Part model, mm, in its own coordinate system. A direction names the side the tool comes from. Give positions to 0.01 mm unless a question says otherwise; leave off trailing zeros. Write each loop counter-clockwise with the first axis right and the second up, starting at its lowest first coordinate (ties: lowest second). Pieces come first, ordered by that corner, then holes. Notation, with made-up numbers: M -7.75,-3.5 L 28.25,-3.5 A25 cw 28.25,13.5 Z; hole C 51.25,-32 d2. An arc over 180 degrees is marked long. Answer as CSV lines item,"result". Start each with the question number.
1) Mould opens along X. For faces 4 (the flat face through (0, 24.3, 2)), 5 (the flat face through (-31, 8, 2)), 6 (the flat face through (-8, -21, 2)) say: pulls with the +X half, pulls with the -X half, needs draft (parallel to the pull), parting line crosses it, or undercut.
2) Pin check, flat tips, straight feed: pin 1 Ø1.6 at (y, z) = (-22.5, 2) entering from -X; pin 2 Ø1 at (y, z) = (8.5, 2.5) entering from +X; pin 3 Ø1.6 at (x, z) = (-9, 1.5) entering from -Y. Stop position of each tip, or through.
3) Wall check: line 1 along X through (y, z) = (-22, 2.9); line 2 along Y through (x, z) = (11, 0.25); line 3 along X through (y, z) = (-5, 1.25). Give the ranges that are in metal, low to high. Write a range as from..to.
4) Slice it at B-B, the plane x = -26. Give the cut face in (y, z), plus the area to 3 significant figures.
5) Tool access for faces 1 (the flat face through (-33, 20, 2)), 2 (the flat face through (33, 4, 2)), 3 (the flat face through (33, -20, 2)): list every direction of +Z, -Z, +X, -X, +Y, -Y with a clear straight run to the whole face (end or side of a thin tool).
6) Slice it at A-A, the plane y = -7. Give the cut face in (x, z), plus the area to 3 significant figures.
```python
from build123d import *

# Parameters (mm, degrees)
ESQUISSE1_W                    = 62
ESQUISSE1_H                    = 42
BOSS_EXTRU_1_DEPTH             = 3.3
ESQUISSE2_W                    = 8
ESQUISSE2_H                    = 3.3
BOSS_EXTRU_2_DEPTH             = 3.3
R_P_TITION_LIN_AIRE1_COUNT     = 2
R_P_TITION_LIN_AIRE1_PITCH     = 16
R_P_TITION_LIN_AIRE1_COL_COUNT = 2
R_P_TITION_LIN_AIRE1_COL_PITCH = 16
SYM_TRIE1_COPY_1_SKETCH_W      = 8
SYM_TRIE1_COPY_1_SKETCH_H      = 3.3
SYM_TRIE1_COPY_1_DEPTH         = 3.3
SYM_TRIE1_COPY_2_SKETCH_W      = 8
SYM_TRIE1_COPY_2_SKETCH_H      = 3.3
SYM_TRIE1_COPY_2_DEPTH         = 3.3
ESQUISSE3_W                    = 3.3
ESQUISSE3_H                    = 8
BOSS_EXTRU_3_DEPTH             = 3.3
R_P_TITION_LIN_AIRE2_COUNT     = 2
R_P_TITION_LIN_AIRE2_PITCH     = 16
R_P_TITION_LIN_AIRE2_COL_COUNT = 2
R_P_TITION_LIN_AIRE2_COL_PITCH = 16
SYM_TRIE2_COPY_1_SKETCH_W      = 3.3
SYM_TRIE2_COPY_1_SKETCH_H      = 8
SYM_TRIE2_COPY_1_DEPTH         = 3.3
SYM_TRIE2_COPY_2_SKETCH_W      = 3.3
SYM_TRIE2_COPY_2_SKETCH_H      = 8
SYM_TRIE2_COPY_2_DEPTH         = 3.3


with BuildPart() as part:
    # Esquisse1 → Boss.-Extru.1 (new body)
    with BuildSketch(Plane.XY):
        Rectangle(ESQUISSE1_W, ESQUISSE1_H)
    extrude(amount=BOSS_EXTRU_1_DEPTH)

    # Esquisse2 → Boss.-Extru.2 (add)
    with BuildSketch(Plane.XY.offset(3.3)):
        with Locations((0, 22.65)):
            Rectangle(ESQUISSE2_W, ESQUISSE2_H)
    boss_extru_2 = extrude(amount=-BOSS_EXTRU_2_DEPTH)

    # Répétition linéaire1: Boss.-Extru.2 ×2
    with Locations(*[(-i * R_P_TITION_LIN_AIRE1_PITCH, 0, 0) for i in range(1, R_P_TITION_LIN_AIRE1_COUNT)]):
        add(boss_extru_2)

    # Répétition linéaire1 col: Boss.-Extru.2 ×2
    with Locations(*[(i * R_P_TITION_LIN_AIRE1_COL_PITCH, 0, 0) for i in range(1, R_P_TITION_LIN_AIRE1_COL_COUNT)]):
        add(boss_extru_2)

    # Symétrie1: Boss.-Extru.2 across plane
    add(boss_extru_2.mirror(Plane.ZX))

    # Symétrie1 copy 1 sketch → Symétrie1 copy 1 (add)
    with BuildSketch(Plane(origin=(-16, 0, 3.3), x_dir=(1, 0, 0), z_dir=(0, 0, 1))):
        with Locations((0, -22.65)):
            Rectangle(SYM_TRIE1_COPY_1_SKETCH_W, SYM_TRIE1_COPY_1_SKETCH_H)
    extrude(amount=-SYM_TRIE1_COPY_1_DEPTH)

    # Symétrie1 copy 2 sketch → Symétrie1 copy 2 (add)
    with BuildSketch(Plane(origin=(16, 0, 3.3), x_dir=(1, 0, 0), z_dir=(0, 0, 1))):
        with Locations((0, -22.65)):
            Rectangle(SYM_TRIE1_COPY_2_SKETCH_W, SYM_TRIE1_COPY_2_SKETCH_H)
    extrude(amount=-SYM_TRIE1_COPY_2_DEPTH)

    # Esquisse3 → Boss.-Extru.3 (add)
    with BuildSketch(Plane.XY.offset(3.3)):
        with Locations((-32.65, 0)):
            Rectangle(ESQUISSE3_W, ESQUISSE3_H)
    boss_extru_3 = extrude(amount=-BOSS_EXTRU_3_DEPTH)

    # Répétition linéaire2: Boss.-Extru.3 ×2
    with Locations(*[(0, i * R_P_TITION_LIN_AIRE2_PITCH, 0) for i in range(1, R_P_TITION_LIN_AIRE2_COUNT)]):
        add(boss_extru_3)

    # Répétition linéaire2 col: Boss.-Extru.3 ×2
    with Locations(*[(0, -i * R_P_TITION_LIN_AIRE2_COL_PITCH, 0) for i in range(1, R_P_TITION_LIN_AIRE2_COL_COUNT)]):
        add(boss_extru_3)

    # Symétrie2: Boss.-Extru.3 across plane
    add(boss_extru_3.mirror(Plane(origin=(0, 0, 0), x_dir=(0, 0, 1), z_dir=(1, 0, 0))))

    # Symétrie2 copy 1 sketch → Symétrie2 copy 1 (add)
    with BuildSketch(Plane(origin=(0, 16, 3.3), x_dir=(-1, 0, 0), z_dir=(0, 0, 1))):
        with Locations((-32.65, 0)):
            Rectangle(SYM_TRIE2_COPY_1_SKETCH_W, SYM_TRIE2_COPY_1_SKETCH_H)
    extrude(amount=-SYM_TRIE2_COPY_1_DEPTH)

    # Symétrie2 copy 2 sketch → Symétrie2 copy 2 (add)
    with BuildSketch(Plane(origin=(0, -16, 3.3), x_dir=(-1, 0, 0), z_dir=(0, 0, 1))):
        with Locations((-32.65, 0)):
            Rectangle(SYM_TRIE2_COPY_2_SKETCH_W, SYM_TRIE2_COPY_2_SKETCH_H)
    extrude(amount=-SYM_TRIE2_COPY_2_DEPTH)


solid = part.part
```
Found:
1,face 4,"needs draft"
1,face 5,"pulls with the -X half"
1,face 6,"undercut"
2,pin 1,"x = -20"
2,pin 2,"x = 31"
2,pin 3,"y = -21"
3,line 1,"-20..-12, -4..4, 12..20"
3,line 2,"-21..21"
3,line 3,"-31..31"
4,outline,"M -21,0 L 21,0 L 21,3.3 L -21,3.3 Z"
4,area,"139 mm²"
5,face 1,"+Z, -Z, -X, +Y"
5,face 2,"+Z, -Z, +X"
5,face 3,"+Z, -Z, +X, -Y"
6,outline,"M -31,0 L 31,0 L 31,3.3 L -31,3.3 Z"
6,area,"205 mm²"
